Can you work these out from the model? Positions are in its coordinate system, mm. A direction names the side the tool comes from. Give positions to 0.01 mm unless a question says otherwise; leave off trailing zeros. Loops run counter-clockwise (first coordinate to the right, second up) from the corner with the lowest first, then second, coordinate; pieces in that order, holes last. Notation, with made-up numbers: (23, -16) - (62, -16) arc R30 cw to (62, 19) - close; hole circle Ø6 at (11, 66). An arc over 180 degrees is marked (long way). Answer in a Markdown table with one row per item.
from build123d import *

# Parameters (mm, degrees)
F1_DEPTH    = 7.5
F2_DEPTH    = 5.5
F3_SIZE2    = 12.5864944677
F3_SIZE     = 15
F5_D        = 3.1
F6_R        = 3
F7_T1_DEPTH = 66.4481797844
F7_T3_DEPTH = 16.376963756
F8_R        = 5


# Not quite as in the source:
# - a fillet or chamfer that OpenCascade refuses, or shapes differently, is made with other operations: its cross-section is extruded or revolved along the edge and cut away or added


with BuildPart() as f1:
    # F0 (on Top) → F1 (new body, symmetric)
    with BuildSketch(Plane.XY):
        Polygon((28, 0), (0, 0), (0, -16), (30.5, -16), (30.5, 0), align=None)
        Polygon((0, 0), (-28, 0), (-30.5, 0), (-30.5, -16), (0, -16), align=None)
    extrude(amount=F1_DEPTH, both=True)

    # F0 (on Top) → F2 (join, symmetric)
    with BuildSketch(Plane.XY):
        with BuildLine():
            Line((-17.5, 3), (-17.5, 5))
            ThreePointArc((-17.5, 5), (-22.1810377062, 1.7052845439), (-23.7029428208, 7.2235332486))
            Line((-23.7029428208, 7.2235332486), (-28, 2))
            Line((-28, 2), (-28, 0))
            Line((-28, 0), (0, 0))
            Line((0, 0), (0, 3))
            Line((0, 3), (-17.5, 3))
        make_face()
        with BuildLine():
            ThreePointArc((-23.7029428208, 7.2235332486), (-22.1810377062, 1.7052845439), (-17.5, 5))
            ThreePointArc((-17.5, 5), (-19.8189622938, 8.2947154561), (-23.7029428208, 7.2235332486))
        make_face()
        with BuildLine():
            ThreePointArc((23.7029428208, 7.2235332486), (19.8189622938, 8.2947154561), (17.5, 5))
            ThreePointArc((17.5, 5), (21, 1.5), (24.5, 5))
            ThreePointArc((24.5, 5), (24.2947154561, 6.1810377062), (23.7029428208, 7.2235332486))
        make_face()
        with BuildLine():
            Line((17.5, 3), (0, 3))
            Line((0, 3), (0, 0))
            Line((0, 0), (28, 0))
            Line((28, 0), (28, 2))
            Line((28, 2), (23.7029428208, 7.2235332486))
            ThreePointArc((23.7029428208, 7.2235332486), (24.2947154561, 6.1810377062), (24.5, 5))
            ThreePointArc((24.5, 5), (21, 1.5), (17.5, 5))
            Line((17.5, 5), (17.5, 3))
        make_face()
    extrude(amount=F2_DEPTH, both=True)

    # F3
    f3_edges = [f1.edges().sort_by_distance(p)[0] for p in [
        (0, -16, -7.5),
    ]]
    f3_side = f1.faces().sort_by_distance((0, -8, -7.5))[0]
    chamfer(f3_edges, length=F3_SIZE, length2=F3_SIZE2, reference=f3_side)

    # F5 (through all)
    with Locations(Plane.XY.offset(5.5)):
        with Locations((-21, 5), (21, 5)):
            Hole(F5_D / 2)

    # F6
    f6_edges = [f1.edges().sort_by_distance(p)[0] for p in [
        (0, -16, 5.086494),
    ]]
    fillet(f6_edges, radius=F6_R)

    # F7: fillet of radius 3 on 3 edges, made by hand

    # F7_s2 → F7_t1 (cut)
    with BuildSketch(Plane.YZ.offset(-33.2240898922)):
        with BuildLine():
            ThreePointArc((-1.8347095698, -6.7995955078), (-0.9762901404, -7.3041789179), (0, -7.5))
            Line((0, -7.5), (-1, -7.5))
            Line((-1, -7.5), (-1.8347095698, -6.7995955078))
        make_face()
    extrude(amount=F7_T1_DEPTH, mode=Mode.SUBTRACT)

    # F7_s4 → F7_t3 (cut)
    with BuildSketch(Plane.XY.offset(-8.188481878)):
        with BuildLine():
            ThreePointArc((-28, 0.9246072488), (-27.8240418195, 1.9369252827), (-27.3168081321, 2.8304928904))
            Line((-27.3168081321, 2.8304928904), (-28, 2))
            Line((-28, 2), (-28, 0.9246072488))
        make_face()
        with BuildLine():
            ThreePointArc((28, 0.9246072488), (27.8240418195, 1.9369252827), (27.3168081321, 2.8304928904))
            Line((27.3168081321, 2.8304928904), (28, 2))
            Line((28, 2), (28, 0.9246072488))
        make_face()
    extrude(amount=F7_T3_DEPTH, mode=Mode.SUBTRACT)

    # F8
    f8_edges = [f1.edges().sort_by_distance(p)[0] for p in [
        (17.5, 3, 0),
        (-17.5, 3, 0),
    ]]
    fillet(f8_edges, radius=F8_R)


solid = f1.part
Q1. On a 3-axis mill with a long thin cutter (end or side, diameter ignored), from which of +Z, -Z, +X, -X, +Y, -Y can I reach the whole of each face in a straight line? I mean faces 4 (the face through (0, 2, 5.5)), 5 (the face through (0, 3, 0)), 6 (the face through (-0.43, -8.47, -1.23)). Say none if no direction works.
Checked values:
| item | result |
|---|---|
| face 4 | +Z, +X, -X, +Y |
| face 5 | +Z, -Z, +Y |
| face 6 | -Z, +X, -X, -Y |
Q2. Imagine slicing it at C-C, the plane z = 0.5. Count the separate pieces of the cut face and the enclosed holes in it, and give its area (3 significant figures).
Checked values:
| item | result |
|---|---|
| separate pieces | 1 |
| enclosed holes | 2 |
| area | 877 mm² |
Q3. Imagine slicing it at B-B, the plane x = -7. Write out the boundary of the cut face in (y, z).
Checked values:
| item | result |
|---|---|
| outline | (-16, 6.49) arc R3 ccw to (-14.93, 4.19) - (-1.83, -6.8) arc R3 ccw to (0, -7.5) - (0, -5.5) - (3, -5.5) - (3, 5.5) - (0, 5.5) - (0, 7.5) - (-16, 7.5) - close |
Q4. If I drill on line 1 (X direction, y = 4.25, z = -4.25); line 2 (Y direction, x = -21, z = -2.25); line 3 (Z direction, x = 10, y = 1.5), over which ranges is the centre line in solid material (lowest first)? Write a range as [from, to].
Checked values:
| item | result |
|---|---|
| line 1 | x = [-26.15, -22.36], [-19.64, -16.35], [16.35, 19.64], [22.36, 26.15] |
| line 2 | y = [-7.26, 3.45], [6.55, 8.5] |
| line 3 | z = [-5.5, 5.5] |
Q5. Imagine slicing it at A-A, the plane x = 21. Write out the boundary of the cut face in (y, z), and give its area (3 significant figures).
Checked values:
| item | result |
|---|---|
| outline | (-16, 6.49) arc R3 ccw to (-14.93, 4.19) - (-1.83, -6.8) arc R3 ccw to (0, -7.5) - (0, -5.5) - (3.45, -5.5) - (3.45, 5.5) - (0, 5.5) - (0, 7.5) - (-16, 7.5) - close; (6.55, -5.5) - (8.5, -5.5) - (8.5, 5.5) - (6.55, 5.5) - close |
| area | 205 mm² |
Q6. If we mould it in two halves opening along Y, with no side actions, what happens to faces 1 (the face through (-25.485, 5.058, 0.077)), 2 (the face through (19.568, 4.406, -0.077)), 3 (the face through (-30.5, -6, 2))? For each: released by +Y, released by -Y, zero draft, split by the parting line, or undercut.
Checked values:
| item | result |
|---|---|
| face 1 | released by +Y |
| face 2 | undercut |
| face 3 | zero draft |
Q7. Imagine slicing it at D-D, the plane y = -3.75. Write out the boundary of the cut face in (x, z).
Checked values:
| item | result |
|---|---|
| outline | (-30.5, -5.19) - (30.5, -5.19) - (30.5, 7.5) - (-30.5, 7.5) - close |
Q8. For pin 1 (4 mm diameter, centred on x = -21, y = 5, fed in from -Z); pin 2 (7.5 mm diameter, centred on x = -15, z = 2, fed in from +Y); pin 3 (1 mm diameter, centred on y = -9.5, z = -1.5, fed in from +X); pin 4 (1 mm diameter, centred on x = 13.5, z = -5.5, fed in from +Y), each with a flat end and sliding along its axis, tell me the tip position at first contact or that it passes through.
Checked values:
| item | result |
|---|---|
| pin 1 | stops at z = -5.5 |
| pin 2 | stops at y = 7.68 |
| pin 3 | passes through |
| pin 4 | stops at y = 3.09 |
